Part model, mm, in its own coordinate system. A direction names the side the tool comes from. Round coordinates to 2 decimals unless told otherwise and drop trailing zeros. Loops run counter-clockwise (first coordinate to the right, second up) from the corner with the lowest first, then second, coordinate; pieces in that order, holes last. Notation, with made-up numbers: M -9.5,38 L 40.5,38 A23 cw 40.5,53 Z; hole C 39.25,42 d3. An arc over 180 degrees is marked long. Put each result on its own line as item: value. Start each with the question number.
```python
from build123d import *

# Parameters (mm, degrees)
SKETCH1_W           = 94.5
SKETCH1_H           = 63.5
SKETCH1_W_2         = 90.5
SKETCH1_H_2         = 59.5
BOSS_EXTRUDE1_DEPTH = 10
SKETCH2_W           = 94.5
SKETCH2_H           = 63.5
BOSS_EXTRUDE2_DEPTH = 2
SKETCH3_W           = 94.5
SKETCH3_H           = 63.5
SKETCH3_W_2         = 76
SKETCH3_H_2         = 3.3
BOSS_EXTRUDE3_DEPTH = 10
SKETCH5_W           = 20
SKETCH5_H           = 2
CUT_EXTRUDE1_DEPTH  = 8
SKETCH6_W           = 2
SKETCH6_H           = 59
CUT_EXTRUDE2_DEPTH  = 6


with BuildPart() as part:
    # Sketch1 → Boss-Extrude1 (new body)
    with BuildSketch(Plane.XY):
        Rectangle(SKETCH1_W, SKETCH1_H)
        Rectangle(SKETCH1_W_2, SKETCH1_H_2, mode=Mode.SUBTRACT)
    extrude(amount=BOSS_EXTRUDE1_DEPTH)

    # Sketch2 → Boss-Extrude2 (add)
    with BuildSketch(Plane.XY):
        Rectangle(SKETCH2_W, SKETCH2_H)
    extrude(amount=BOSS_EXTRUDE2_DEPTH)

    # Sketch3 → Boss-Extrude3 (add)
    with BuildSketch(Plane(origin=(0, 0, 0), x_dir=(-1, 0, 0), z_dir=(0, 0, -1))):
        Rectangle(SKETCH3_W, SKETCH3_H)
        Rectangle(SKETCH3_W_2, SKETCH3_H_2, mode=Mode.SUBTRACT)
    extrude(amount=BOSS_EXTRUDE3_DEPTH)

    # Sketch5 → Cut-Extrude1 (cut)
    with BuildSketch(Plane.XY.offset(10)):
        with Locations((-35.25, -30.75)):
            Rectangle(SKETCH5_W, SKETCH5_H)
    extrude(amount=-CUT_EXTRUDE1_DEPTH, mode=Mode.SUBTRACT)

    # Sketch6 → Cut-Extrude2 (cut)
    with BuildSketch(Plane.XY.offset(10)):
        with Locations((46.25, 0.25)):
            Rectangle(SKETCH6_W, SKETCH6_H)
    extrude(amount=-CUT_EXTRUDE2_DEPTH, mode=Mode.SUBTRACT)


solid = part.part
```
1. Cut at C-C, the plane z = -4.5. Give the cut face in (x, y).
2. Cut at D-D, the plane y = 23. Give the cut face in (x, z).
3. Wall check: L1, parallel to Y at x = 36.5, z = -5; L2, parallel to Y at x = 30, z = 2.75; L3, parallel to X at y = -14.5, z = 3. Give the ranges that are in metal, low to high.
4. Drop flat-ended pins along their axis: pin 1 (6 mm diameter, centred on x = 2, y = 3, fed in from +Z); pin 2 (1 mm diameter, centred on x = 46, y = 4.5, fed in from +Z). Give the stop position or say it passes through.
5. Cut at A-A, the plane z = 8. Give the cut face in (x, y), and give its area (3 significant figures).
6. Which spindle directions (+Z, -Z, +X, -X, +Y, -Y) get a long thin tool onto all of the face, cutting with end or side? Do faces 5 (the flat face through (-47.25, 0, 0)), 6 (the flat face through (46, 1, 4)), 7 (the flat face through (-38, 0, -5)), 8 (the flat face through (-45.25, -1, 6)), 9 (the flat face through (0, 29.75, 6)). Say none if no direction does.
7. Mould opens along X. For faces 1 (the flat face through (-21, 31, 10)), 2 (the flat face through (47.25, 0, -4)), 3 (the flat face through (-1, -1, 2)), 4 (the flat face through (1, -1.65, -5)) say: released by +X, released by -X, zero draft, split by the parting line, or undercut.
8. Cut at B-B, the plane x = 13. Give the cut face in (y, z), and give its area (3 significant figures).
Results list:
1. outline: M -47.25,-31.75 L 47.25,-31.75 L 47.25,31.75 L -47.25,31.75 Z; hole M -38,-1.65 L 38,-1.65 L 38,1.65 L -38,1.65 Z
2. outline: M -47.25,-10 L 47.25,-10 L 47.25,4 L 45.25,4 L 45.25,2 L -45.25,2 L -45.25,10 L -47.25,10 Z
3. L1: y = -31.75 to -1.65, 1.65 to 31.75
3. L2: y = -31.75 to -29.75, 29.75 to 31.75
3. L3: x = -47.25 to -45.25, 45.25 to 47.25
4. pin 1: stops at z = 2
4. pin 2: stops at z = 4
5. outline: M -47.25,-31.75 L -45.25,-31.75 L -45.25,29.75 L 47.25,29.75 L 47.25,31.75 L -47.25,31.75 Z; M -25.25,-31.75 L 47.25,-31.75 L 47.25,-29.25 L 45.25,-29.25 L 45.25,-29.75 L -25.25,-29.75 Z
5. area: 458 mm^2
6. face 5: +Z, -Z, -X, +Y, -Y
6. face 6: +Z, +X
6. face 7: -Z
6. face 8: +Z, -Y
6. face 9: +Z
7. face 1: zero draft
7. face 2: released by +X
7. face 3: undercut
7. face 4: undercut
8. outline: M -31.75,-10 L -1.65,-10 L -1.65,0 L 1.65,0 L 1.65,-10 L 31.75,-10 L 31.75,10 L 29.75,10 L 29.75,2 L -29.75,2 L -29.75,10 L -31.75,10 Z
8. area: 761 mm^2
